CAD build for the part. Positions are in the model's coordinates, mm. Give positions to 0.01 mm unless a question says otherwise; leave off trailing zeros. Order: outer loops, then holes, each group sorted by start corner. A loop starts at its lowest first (then second) coordinate and runs counter-clockwise, first axis right, second up. Notation, with made-up numbers: (-17, 54) -> (27, 54) arc R27 cw to (27, 85) -> close; hole circle Ø2 at (81, 41). An arc over 180 degrees is marked (long way). Use one line per item in the form item = value. Start each with the question number.
1) Cut at B-B, the plane x = -48.5. Give the cut face in (y, z).
2) Drop a flat-ended pin along its axis: P1, Ø4.5, axis at x = -78.52, z = 77.25, coming from the -Y side. Give the stop position or say it passes through.
3) Mould opens along Z. For faces 1 (the face through (-59, 5, 123.5)), 2 (the face through (-59, 5, -51.5)), 3 (the face through (-82.5, 5, 8)), 4 (the face through (47.5, 5, 37)) say: pulls with the +Z half, pulls with the -Z half, needs draft (parallel to the pull), parting line crosses it, or undercut.
4) Cut at C-C, the plane y = 2.75. State how many separate pieces and enclosed holes the cut face has, and give its area (3 significant figures).
5) Cut at A-A, the plane x = 30.5. Give the cut face in (y, z).
6) Probe line 1 (Z direction, x = 12, y = 2); line 2 (Z direction, x = -8, y = 3.5); line 3 (X direction, y = 5.75, z = 116). List the from-to ranges inside material, lowest first.
from build123d import *

# Parameters (mm, degrees)
SKETCH_1_W      = 210
SKETCH_1_H      = 175
SKETCH_1_R      = 1.5
SKETCH_1_R_2    = 2
EXTRUDE_1_DEPTH = 10


with BuildPart() as part:
    # Эскиз1 → Бобышка-Вытянуть1 (new body)
    with BuildSketch(Plane(origin=(0, 0, 0), x_dir=(1, 0, 0), z_dir=(0, 1, 0))):
        with Locations((-57.5, -36)):
            Rectangle(SKETCH_1_W, SKETCH_1_H)
        with Locations(Location((-5.5, 15.5, 0), (0, 0, 270))):
            Circle(SKETCH_1_R, mode=Mode.SUBTRACT)
        with Locations(Location((5.5, 15.5, 0), (0, 0, 270))):
            Circle(SKETCH_1_R, mode=Mode.SUBTRACT)
        with Locations(Location((-5.5, -15.5, 0), (0, 0, 270))):
            Circle(SKETCH_1_R, mode=Mode.SUBTRACT)
        with Locations(Location((5.5, -15.5, 0), (0, 0, 270))):
            Circle(SKETCH_1_R, mode=Mode.SUBTRACT)
        with Locations(Location((-36.5, -40.5, 0), (0, 0, 270))):
            Circle(SKETCH_1_R, mode=Mode.SUBTRACT)
        with Locations(Location((-36.5, -113.5, 0), (0, 0, 270))):
            Circle(SKETCH_1_R, mode=Mode.SUBTRACT)
        with Locations(Location((-144.5, 40, 0), (0, 0, 270))):
            Circle(SKETCH_1_R, mode=Mode.SUBTRACT)
        with Locations(Location((-79.5, 2.5, 0), (0, 0, 270))):
            Circle(SKETCH_1_R_2, mode=Mode.SUBTRACT)
        with Locations(Location((-142.5, -15.5, 0), (0, 0, 270))):
            Circle(SKETCH_1_R_2, mode=Mode.SUBTRACT)
        with Locations(Location((-18.5, -40.5, 0), (0, 0, 270))):
            Circle(SKETCH_1_R, mode=Mode.SUBTRACT)
        with Locations(Location((21.5, -40.5, 0), (0, 0, 270))):
            Circle(SKETCH_1_R, mode=Mode.SUBTRACT)
        with Locations(Location((-155, 44, 0), (0, 0, 270))):
            Circle(SKETCH_1_R_2, mode=Mode.SUBTRACT)
        with Locations(Location((40, 44, 0), (0, 0, 270))):
            Circle(SKETCH_1_R_2, mode=Mode.SUBTRACT)
        with Locations(Location((40, -116, 0), (0, 0, 270))):
            Circle(SKETCH_1_R_2, mode=Mode.SUBTRACT)
        with Locations(Location((-155, -116, 0), (0, 0, 270))):
            Circle(SKETCH_1_R_2, mode=Mode.SUBTRACT)
        with Locations(Location((-78.518280062, -77.24520536, 0), (0, 0, 270))):
            Circle(SKETCH_1_R_2, mode=Mode.SUBTRACT)
        Polygon((-13.5, 13), (-28, 12), (-41.5, 12), (-41.5, 13), (-62.5, 13), (-62.5, -89), (-41.5, -89), (-41.5, -108.5), (-31.5, -108.5), (-31.5, -99), (18.5, -99), (18.5, -55), (-31.5, -55), (-31.5, -45.5), (-41.5, -45.5), (-41.5, -12), (-28, -12), (-13.5, -13), (9.5, -13), (9.5, -20), (37.5, -20), (37.5, 20), (9.5, 20), (9.5, 13), align=None, mode=Mode.SUBTRACT)
        with BuildLine():
            Line((-82.5, 17.5), (-82.5, 14.5))
            Line((-82.5, 14.5), (-76.5, 14.5))
            ThreePointArc((-76.5, 14.5), (-72.5, 10.5), (-76.5, 6.5))
            Line((-76.5, 6.5), (-82.5, 6.5))
            Line((-82.5, 6.5), (-82.5, -22.5))
            Line((-82.5, -22.5), (-139.5, -22.5))
            Line((-139.5, -22.5), (-139.5, 17.5))
            Line((-139.5, 17.5), (-82.5, 17.5))
        make_face(mode=Mode.SUBTRACT)
    extrude(amount=EXTRUDE_1_DEPTH)


solid = part.part
Result:
q1.outline = (0, -51.5) -> (10, -51.5) -> (10, -13) -> (0, -13) -> close; (0, 89) -> (10, 89) -> (10, 123.5) -> (0, 123.5) -> close
q2.P1 = 0
q3.face_1 = pulls with the +Z half
q3.face_2 = pulls with the -Z half
q3.face_3 = undercut
q3.face_4 = needs draft
q4.separate_pieces = 1
q4.enclosed_holes = 18
q4.area = 26,900 mm²
q5.outline = (0, -51.5) -> (10, -51.5) -> (10, -20) -> (0, -20) -> close; (0, 20) -> (10, 20) -> (10, 123.5) -> (0, 123.5) -> close
q6.line_1 = -51.5 to -20, 20 to 55, 99 to 123.5
q6.line_2 = -51.5 to -13, 13 to 55, 99 to 123.5
q6.line_3 = -162.5 to -157, -153 to 38, 42 to 47.5
